from build123d import *

# Parameters (mm, degrees)
SKETCH3_R   = 2.5
SKETCH3_W   = 16
SKETCH3_H   = 16
LASER_DEPTH = 2


with BuildPart() as part:
    # Sketch3 → Laser (new body)
    with BuildSketch(Plane(origin=(0, 0, 0), x_dir=(1, 0, 0), z_dir=(0, 1, 0))):
        with BuildLine():
            Line((-94.691051343, -6.582969065), (-21.663792567, 32.211956563))
            ThreePointArc((-21.663792567, 32.211956563), (-18.18495221, 33.546260198), (-14.486734177, 34))
            Line((-14.486734177, 34), (157, 34))
            Line((157, 34), (157, -80.984375239))
            Line((157, -80.984375239), (27.245097002, -82.002060753))
            ThreePointArc((27.245097002, -82.002060753), (-3.897107576, -90.097611519), (-27.500192145, -111.966979298))
            Line((-27.500192145, -111.966979298), (-50.631086639, -93.38167756))
            ThreePointArc((-50.631086639, -93.38167756), (-55.49562639, -87.852512852), (-58.20502519, -81.004552024))
            ThreePointArc((-58.20502519, -81.004552024), (-60.798796423, -71.823881458), (-64.66560314, -63.102633435))
            Line((-64.66560314, -63.102633435), (-94.691051343, -6.582969065))
        make_face()
        with Locations(Location((-22.393572022, 24.996840478, 0), (0, 0, 270))):
            Circle(SKETCH3_R, mode=Mode.SUBTRACT)
        with Locations(Location((-6.470173498, -4.977237981, 0), (0, 0, 270))):
            Circle(SKETCH3_R, mode=Mode.SUBTRACT)
        with Locations(Location((-36.444251957, -20.900636504, 0), (0, 0, 270))):
            Circle(SKETCH3_R, mode=Mode.SUBTRACT)
        with Locations(Location((-52.367650481, 9.073441955, 0), (0, 0, 270))):
            Circle(SKETCH3_R, mode=Mode.SUBTRACT)
        with Locations((9, -10)):
            Rectangle(SKETCH3_W, SKETCH3_H, mode=Mode.SUBTRACT)
        with Locations((9, 9)):
            Rectangle(SKETCH3_W, SKETCH3_H, mode=Mode.SUBTRACT)
        with Locations((28, 11)):
            Rectangle(SKETCH3_W, SKETCH3_H, mode=Mode.SUBTRACT)
        with Locations((47, 23)):
            Rectangle(SKETCH3_W, SKETCH3_H, mode=Mode.SUBTRACT)
        with Locations((66, 18)):
            Rectangle(SKETCH3_W, SKETCH3_H, mode=Mode.SUBTRACT)
        with Locations((85, 9)):
            Rectangle(SKETCH3_W, SKETCH3_H, mode=Mode.SUBTRACT)
        with Locations((104, 6)):
            Rectangle(SKETCH3_W, SKETCH3_H, mode=Mode.SUBTRACT)
        with Locations((123, 6)):
            Rectangle(SKETCH3_W, SKETCH3_H, mode=Mode.SUBTRACT)
        with Locations((146, 1.25)):
            Rectangle(SKETCH3_W, SKETCH3_H, mode=Mode.SUBTRACT)
        with Locations((146, -65.25)):
            Rectangle(SKETCH3_W, SKETCH3_H, mode=Mode.SUBTRACT)
        with Locations((28, -8)):
            Rectangle(SKETCH3_W, SKETCH3_H, mode=Mode.SUBTRACT)
        with Locations((47, 4)):
            Rectangle(SKETCH3_W, SKETCH3_H, mode=Mode.SUBTRACT)
        with Locations((66, -1)):
            Rectangle(SKETCH3_W, SKETCH3_H, mode=Mode.SUBTRACT)
        with Locations((85, -10)):
            Rectangle(SKETCH3_W, SKETCH3_H, mode=Mode.SUBTRACT)
        with Locations((104, -13)):
            Rectangle(SKETCH3_W, SKETCH3_H, mode=Mode.SUBTRACT)
        with Locations((123, -13)):
            Rectangle(SKETCH3_W, SKETCH3_H, mode=Mode.SUBTRACT)
        with Locations((9, -29)):
            Rectangle(SKETCH3_W, SKETCH3_H, mode=Mode.SUBTRACT)
        with Locations((28, -27)):
            Rectangle(SKETCH3_W, SKETCH3_H, mode=Mode.SUBTRACT)
        with Locations((47, -15)):
            Rectangle(SKETCH3_W, SKETCH3_H, mode=Mode.SUBTRACT)
        with Locations((66, -20)):
            Rectangle(SKETCH3_W, SKETCH3_H, mode=Mode.SUBTRACT)
        with Locations((85, -29)):
            Rectangle(SKETCH3_W, SKETCH3_H, mode=Mode.SUBTRACT)
        with Locations((104, -32)):
            Rectangle(SKETCH3_W, SKETCH3_H, mode=Mode.SUBTRACT)
        with Locations((123, -32)):
            Rectangle(SKETCH3_W, SKETCH3_H, mode=Mode.SUBTRACT)
        with Locations((9, -48)):
            Rectangle(SKETCH3_W, SKETCH3_H, mode=Mode.SUBTRACT)
        with Locations((28, -46)):
            Rectangle(SKETCH3_W, SKETCH3_H, mode=Mode.SUBTRACT)
        with Locations((47, -34)):
            Rectangle(SKETCH3_W, SKETCH3_H, mode=Mode.SUBTRACT)
        with Locations((66, -39)):
            Rectangle(SKETCH3_W, SKETCH3_H, mode=Mode.SUBTRACT)
        with Locations((85, -48)):
            Rectangle(SKETCH3_W, SKETCH3_H, mode=Mode.SUBTRACT)
        Polygon((-88.288511049, -12.240484229), (-74.158594957, -4.734122178), (-66.652232907, -18.86403827), (-80.782148999, -26.370400321), align=None, mode=Mode.SUBTRACT)
        with Locations((13.75, -71)):
            Rectangle(SKETCH3_W, SKETCH3_H, mode=Mode.SUBTRACT)
        with Locations((108.75, -51)):
            Rectangle(SKETCH3_W, SKETCH3_H, mode=Mode.SUBTRACT)
        with Locations((108.75, -70)):
            Rectangle(SKETCH3_W, SKETCH3_H, mode=Mode.SUBTRACT)
        Polygon((-65.244790023, -21.513397538), (-79.374706115, -29.019759588), (-71.868344064, -43.14967568), (-57.738427972, -35.64331363), align=None, mode=Mode.SUBTRACT)
        Polygon((-53.68162582, -36.885230013), (-39.551709728, -29.378867962), (-32.045347678, -43.508784054), (-46.17526377, -51.015146105), align=None, mode=Mode.SUBTRACT)
        Polygon((-27.988545526, -44.750700437), (-13.858629434, -37.244338387), (-6.352267384, -51.374254479), (-20.482183476, -58.880616529), align=None, mode=Mode.SUBTRACT)
        Polygon((-30.637904794, -46.158143322), (-44.767820886, -53.664505372), (-37.261458835, -67.794421464), (-23.131542743, -60.288059414), align=None, mode=Mode.SUBTRACT)
        Polygon((-47.417180153, -55.071948256), (-61.547096245, -62.578310307), (-54.040734195, -76.708226399), (-39.910818103, -69.201864348), align=None, mode=Mode.SUBTRACT)
        Polygon((-34.248075282, -82.171885463), (-44.269669774, -94.644561352), (-31.796993885, -104.666155844), (-21.775399393, -92.193479955), align=None, mode=Mode.SUBTRACT)
        Polygon((-25.21699676, -74.701037634), (-11.087080668, -67.194675584), (-3.580718618, -81.324591676), (-17.71063471, -88.830953726), align=None, mode=Mode.SUBTRACT)
        Polygon((-40.237051061, 5.359879008), (-26.107134969, 12.866241058), (-18.600772918, -1.263675034), (-32.73068901, -8.770037084), align=None, mode=Mode.SUBTRACT)
    extrude(amount=-LASER_DEPTH)


solid = part.part
Geometry: final body of the model. Coordinates: model frame, mm. A direction names the side the tool comes from. Round coordinates to 2 decimals unless told otherwise and drop trailing zeros. Order: outer loops, then holes, each group sorted by start corner. A loop starts at its lowest first (then second) coordinate and runs counter-clockwise, first axis right, second up. Notation, with made-up numbers: (-28, -36.75) -> (16, -36.75) arc R17 cw to (16, -17.75) -> close; hole circle Ø4 at (-1.5, 28). An arc over 180 degrees is marked (long way). Put each result on its own line as item: value. Start each with the question number.
Q1. Pull-direction query (Z, two-part tool) for faces 1 (the flat face through (-33.27, -0.99, -9.06)), 2 (the cylindrical face through (-3.5, -0.99, 89.88)), 3 (the flat face through (-58.69, -0.99, -12.54)); classes: +Z half, -Z half, draft (parallel to the pull), parting line (faces both ways), or undercut.
Q2. Reachability of faces 4 (the flat face through (-35.851, -0.986, 36.345)), 5 (the flat face through (-79.468, -0.986, 35.238)) from +Z, -Z, +X, -X, +Y, -Y: full face, straight path, thin tool, end or side. Return the list, or none.
Q3. First-contact query: pin 1 (0.6 mm diameter, centred on x = 8, y = -1, fed in from +Z); pin 2 (1 mm diameter, centred on y = -1, z = 89, fed in from +X); pin 3 (1 mm diameter, centred on x = 15, y = -1, fed in from +Z). Flat tips, straight axial feed; report the tip coordinate or a pass-through.
Q4. Section C-C on y = -0.45. Give the number of separate pieces and of enclosed holes in the cut face, and give its area (3 significant figures).
Q5. Section A-A on z = 85. Return the cut outline in (x, y).
Q6. Section B-B on x = 104. Return the cut outline in (y, z).
Q7. Line query: probe 1 along Z at (x, y) = (114.5, -1.6); probe 2 along Z at (x, y) = (-32, -1.45); probe 3 along Z at (x, y) = (65.5, -1.4). Output: solid intervals per line, ascending.
Ans:
1. face 1: undercut
1. face 2: +Z half
1. face 3: -Z half
2. face 4: +Y, -Y
2. face 5: +Z, -X, +Y, -Y
3. pin 1: stops at z = 85.13
3. pin 2: stops at x = -0.79
3. pin 3: stops at z = 83.35
4. separate pieces: 1
4. enclosed holes: 44
4. area: 16,800 mm2
5. outline: (-56.96, -2) -> (-36.52, -2) -> (-36.52, 0) -> (-56.96, 0) -> close; (-30.73, -2) -> (-19.75, -2) -> (-19.75, 0) -> (-30.73, 0) -> close; (-10.5, -2) -> (8.1, -2) -> (8.1, 0) -> (-10.5, 0) -> close
6. outline: (-2, -34) -> (0, -34) -> (0, -14) -> (-2, -14) -> close; (-2, 2) -> (0, 2) -> (0, 5) -> (-2, 5) -> close; (-2, 21) -> (0, 21) -> (0, 24) -> (-2, 24) -> close; (-2, 40) -> (0, 40) -> (0, 43) -> (-2, 43) -> close; (-2, 59) -> (0, 59) -> (0, 62) -> (-2, 62) -> close; (-2, 78) -> (0, 78) -> (0, 81.4) -> (-2, 81.4) -> close
7. probe 1: z = -34 to 43, 59 to 62, 78 to 81.32
7. probe 2: z = -26.72 to -9.74, 8.38 to 46.88, 65 to 83.98, 104.5 to 108.35
7. probe 3: z = -34 to -26, -10 to -7, 9 to 12, 28 to 31, 47 to 81.7
